```python
from build123d import *

# Parameters (mm, degrees)
BOSS_EXTRUDE1_DEPTH = 10
FILLET1_R           = 0.3
FILLET2_R           = 0.2
TAPPED_HOLE1_D      = 4.134


with BuildPart() as part:
    # Sketch1 → Boss-Extrude1 (new body)
    with BuildSketch(Plane(origin=(-5, 0, 0), x_dir=(0, 0, -1), z_dir=(1, 0, 0))):
        with BuildLine():
            Line((2.5, -4.1), (-2.5, -4.1))
            Line((-2.5, -4.1), (-4.94636223, -1.177635916))
            ThreePointArc((-4.94636223, -1.177635916), (-4.978394171, -0.932676469), (-4.77, -0.8))
            Line((-4.77, -0.8), (-2.9, -0.8))
            Line((-2.9, -0.8), (-2.9, 0))
            Line((-2.9, 0), (2.9, 0))
            Line((2.9, 0), (2.9, -0.8))
            Line((2.9, -0.8), (4.77, -0.8))
            ThreePointArc((4.77, -0.8), (4.978394171, -0.932676469), (4.94636223, -1.177635916))
            Line((4.94636223, -1.177635916), (2.5, -4.1))
        make_face()
    extrude(amount=BOSS_EXTRUDE1_DEPTH)

    # Fillet1
    fillet1_edges = [part.edges().sort_by_distance(p)[0] for p in [
        (0, -4.1, -2.5),
        (0, -4.1, 2.5),
    ]]
    fillet(fillet1_edges, radius=FILLET1_R)

    # Fillet2
    fillet2_edges = [part.edges().sort_by_distance(p)[0] for p in [
        (0, 0, 2.9),
        (0, 0, -2.9),
    ]]
    fillet(fillet2_edges, radius=FILLET2_R)

    # Tapped Hole1 (through all)
    with Locations(Plane(origin=(0, 0, 0), x_dir=(1, 0, 0), z_dir=(0, 1, 0))):
        with Locations((0, 0)):
            Hole(TAPPED_HOLE1_D / 2)


solid = part.part
```
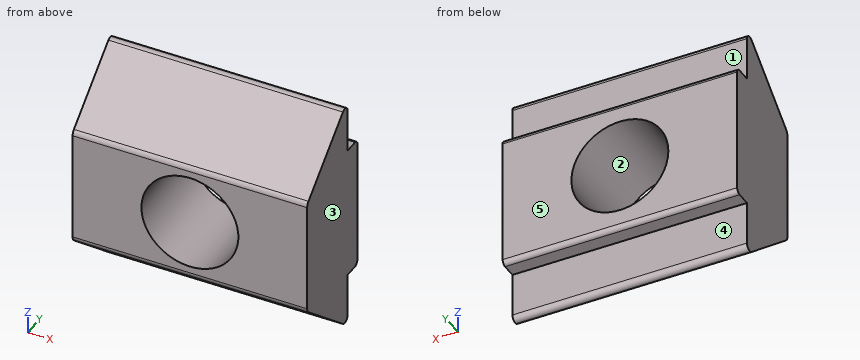
The model under review builds one solid part; all positions refer to its coordinate system, in mm. Face numbers are marked on the shaded views. A direction names the side the tool comes from. Round coordinates to 2 decimals unless told otherwise and drop trailing zeros. Write each loop counter-clockwise with the first axis right and the second up, starting at its lowest first coordinate (ties: lowest second). Pieces come first, ordered by that corner, then holes. Notation, with made-up numbers: (-21, 1) - (2, 1) arc R23 cw to (2, 26) - close; hole circle Ø5 at (27.25, 78.25). An arc over 180 degrees is marked (long way). One line per question, with ' | ' between items.
Item 1: Add section A-A, the plane x = 0. Give the boundary of the cut face in (y, z).
Resolved:
outline: (-4.1, -2.36) arc R0.3 ccw to (-3.99, -2.59) - (-1.18, -4.95) arc R0.23 ccw to (-0.8, -4.77) - (-0.8, -2.9) - (-0.2, -2.9) arc R0.2 ccw to (0, -2.7) - (0, -2.07) - (-4.1, -2.07) - close; (-4.1, 2.07) - (0, 2.07) - (0, 2.7) arc R0.2 ccw to (-0.2, 2.9) - (-0.8, 2.9) - (-0.8, 4.77) arc R0.23 ccw to (-1.18, 4.95) - (-3.99, 2.59) arc R0.3 ccw to (-4.1, 2.36) - close
Item 2: To check wall thickness, follow probe 1 along Z at (x, y) = (0.75, -0.65); probe 2 along Z at (x, y) = (0, -1.5); probe 3 along Y at (x, z) = (3.5, 3.25). State the ranges of each line that lie inside material, in increasing order.
Resolved:
probe 1: z = -2.9 to -1.93, 1.93 to 2.9 | probe 2: z = -4.68 to -2.07, 2.07 to 4.68 | probe 3: y = -3.2 to -0.8
Item 3: For the marked faces 4 and 5, list the 3-axis set-ups (+Z, -Z, +X, -X, +Y, -Y) from which the entire face can be reached by the end or side of a thin tool; tool diameter is ignored.
Resolved:
face 4: -Z, +X, -X, +Y | face 5: +Z, -Z, +X, -X, +Y
Item 4: For P1, Ø1, axis at x = 0, y = -2, coming from the +Z side; P2, Ø1.5, axis at x = -1.5, z = -4, coming from the +Y side; P3, Ø0.5, axis at x = 2, y = -0.5, coming from the +Z side, all flat-tipped, find the tip position at first contact; note any pin that passes through.
Resolved:
P1: stops at z = 4.68 | P2: stops at y = -0.8 | P3: stops at z = 2.9
Item 5: Add section B-B, the plane z = 0. Give the boundary of the cut face in (x, y), then the cut area to 3 significant figures.
Resolved:
outline: (-5, -4.1) - (-2.07, -4.1) - (-2.07, 0) - (-5, 0) - close; (2.07, -4.1) - (5, -4.1) - (5, 0) - (2.07, 0) - close | area: 24.1 mm2
Item 6: Add section C-C, the plane x = 2.75. Give the boundary of the cut face in (y, z), then the cut area to 3 significant figures.
Resolved:
outline: (-4.1, -2.36) arc R0.3 ccw to (-3.99, -2.59) - (-1.18, -4.95) arc R0.23 ccw to (-0.8, -4.77) - (-0.8, -2.9) - (-0.2, -2.9) arc R0.2 ccw to (0, -2.7) - (0, 2.7) arc R0.2 ccw to (-0.2, 2.9) - (-0.8, 2.9) - (-0.8, 4.77) arc R0.23 ccw to (-1.18, 4.95) - (-3.99, 2.59) arc R0.3 ccw to (-4.1, 2.36) - close | area: 30.1 mm2
Item 7: Add section D-D, the plane y = -2. Give the boundary of the cut face in (x, z), then the cut area to 3 significant figures.
Resolved:
outline: (-5, -4.26) - (5, -4.26) - (5, 4.26) - (-5, 4.26) - close; hole circle Ø4.13 at (0, 0) | area: 71.7 mm2
Item 8: The part is to be moulded in two halves that separate along X. For the marked faces 1, 2 and 3, say which applies: pulls with the +X half, pulls with the -X half, needs draft (parallel to the pull), parting line crosses it, or undercut.
Resolved:
face 1: needs draft | face 2: undercut | face 3: pulls with the +X half
